from build123d import *

# Parameters (mm, degrees)
F0_W     = 469.9
F0_H     = 406.4
F1_DEPTH = 19.05
F3_D     = 15.0114
F3_DEPTH = 14.224
F3_TIP   = 4.5098795482
F5_D     = 8.001
F5_DEPTH = 25.4
F5_TIP   = 2.4037429064
F7_D     = 8.001
F7_DEPTH = 25.4
F7_TIP   = 2.4037429064
F9_D     = 8.001
F9_DEPTH = 25.4
F9_TIP   = 2.4037429064


with BuildPart() as f1:
    # F0 (on Top) → F1 (new body)
    with BuildSketch(Plane.XY):
        Rectangle(F0_W, F0_H)
    extrude(amount=F1_DEPTH)

    # F3
    with Locations(Plane(origin=(0, 0, 0), x_dir=(1, 0, 0), z_dir=(0, 0, -1))):
        with Locations((-211.074, 152.4), (-211.074, 0), (-211.074, -152.4), (-184.15, -179.324), (0, -179.324), (184.15, -179.324), (211.074, -152.4), (211.074, 0), (211.074, 152.4)):
            Hole(F3_D / 2, depth=F3_DEPTH)
            with Locations((0, 0, -(F3_DEPTH + F3_TIP / 2))):  # 118° drill point
                Cone(0, F3_D / 2, F3_TIP, mode=Mode.SUBTRACT)

    # F5
    with Locations(Plane.YZ.offset(234.95)):
        with Locations((-152.4, 9.525), (0, 9.525), (152.4, 9.525)):
            Hole(F5_D / 2, depth=F5_DEPTH)
            with Locations((0, 0, -(F5_DEPTH + F5_TIP / 2))):  # 118° drill point
                Cone(0, F5_D / 2, F5_TIP, mode=Mode.SUBTRACT)

    # F7
    with Locations(Plane(origin=(0, 203.2, 0), x_dir=(-1, 0, 0), z_dir=(0, 1, 0))):
        with Locations((-184.15, 9.525), (0, 9.525), (184.15, 9.525)):
            Hole(F7_D / 2, depth=F7_DEPTH)
            with Locations((0, 0, -(F7_DEPTH + F7_TIP / 2))):  # 118° drill point
                Cone(0, F7_D / 2, F7_TIP, mode=Mode.SUBTRACT)

    # F9
    with Locations(Plane(origin=(-234.95, 0, 0), x_dir=(0, -1, 0), z_dir=(-1, 0, 0))):
        with Locations((-152.4, 9.525), (0, 9.525), (152.4, 9.525)):
            Hole(F9_D / 2, depth=F9_DEPTH)
            with Locations((0, 0, -(F9_DEPTH + F9_TIP / 2))):  # 118° drill point
                Cone(0, F9_D / 2, F9_TIP, mode=Mode.SUBTRACT)


solid = f1.part
Geometry check sheet. Reference: the model listing, model coordinates, mm. A direction names the side the tool comes from. Coordinates: 2 decimals unless noted, no trailing zeros. One line per item, written item: value.
(1) Release check for a two-part mould opening along X. For faces 3 (the face through (-183.45, 178.22, 17.95)), 4 (the face through (-234.95, -3, 14)), 5 (the face through (211.675, -151.244, 17.951)), 6 (the face through (-3, 203.2, 14)) record: +X half, -X half, draft (parallel to the pull), parting line (faces both ways), or undercut.
Data:
face 3: undercut
face 4: -X half
face 5: undercut
face 6: draft
(2) Access from +Z, -Z, +X, -X, +Y, -Y to the whole of each face (thin tool, end or side, straight path). Record for faces 1 (the face through (0.977, 171.882, 7.212)), 2 (the face through (234.95, -3, 14)).
Data:
face 1: -Z
face 2: +Z, -Z, +X, +Y, -Y
(3) Depth check by flat-ended pin: pin 1 Ø5 at (y, z) = (0, 9.525) entering from -X; pin 2 Ø13.5 at (x, y) = (-211.074, 152.4) entering from -Z; pin 3 Ø7 at (x, z) = (184.15, 9.525) entering from +Y. Enter the tip coordinate at first touch or a pass-through.
Data:
pin 1: stops at x = -204
pin 2: stops at z = 14.68
pin 3: stops at y = 172.68
(4) Thickness scan on probe 1 along X at (y, z) = (152.4, 3.5); probe 2 along Y at (x, z) = (212, 10); probe 3 along Z at (x, y) = (184.15, 199.5). Record the ranges inside material, lowest first. Write a range as from..to.
Data:
probe 1: x = -234.95..-218.58, -203.57..203.57, 218.58..234.95
probe 2: y = -203.2..-159.85, -144.95..-7.45, 7.45..144.95, 159.85..203.2
probe 3: z = 0..5.52, 13.53..19.05
